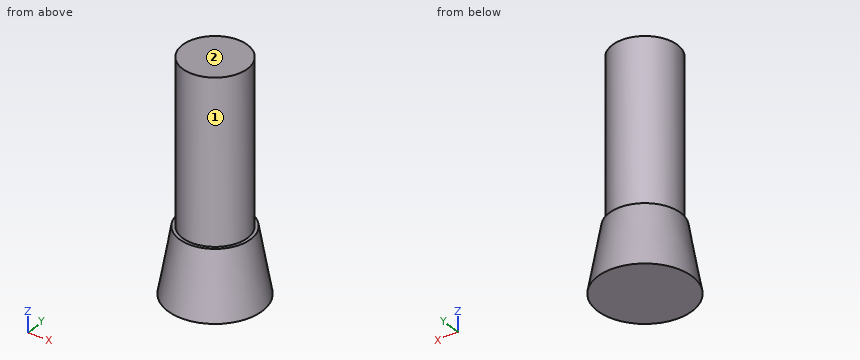
```python
from build123d import *

# Parameters (mm, degrees)
F0_R     = 12.7
F1_DEPTH = 88.9
F0_R_2   = 19.05
F2_DEPTH = 25.4


# Not quite as in the source:
# - a fillet or chamfer that OpenCascade refuses, or shapes differently, is made with other operations: its cross-section is extruded or revolved along the edge and cut away or added


with BuildPart() as f1:
    # F0 (on Top) → F1 (new body)
    with BuildSketch(Plane.XY):
        Circle(F0_R)
    extrude(amount=F1_DEPTH)

    # F0 (on Top) → F2 (join)
    with BuildSketch(Plane.XY):
        Circle(F0_R_2)
        Circle(F0_R, mode=Mode.SUBTRACT)
    extrude(amount=F2_DEPTH)

    # F3: chamfer of 5.08 x 28.8101116437 on 1 edges, made by hand

    # F3_s1 → F3_t2 (revolve, cut)
    with BuildSketch(Plane.XZ):
        Polygon((13.97, 25.4), (19.05, -3.4101116437), (19.05, 25.4), align=None)
    revolve(axis=Axis((0, 0, 25.4), (0, 0, 1)), mode=Mode.SUBTRACT)


solid = f1.part
```
For this review, take the finished solid that the model builds, in its own axes (mm). Face numbers are marked on the shaded views. A direction names the side the tool comes from. Round coordinates to 2 decimals unless told otherwise and drop trailing zeros. Write each loop counter-clockwise with the first axis right and the second up, starting at its lowest first coordinate (ties: lowest second). Pieces come first, ordered by that corner, then holes. Notation, with made-up numbers: (72, 30.5) -> (108, 30.5) arc R16 ccw to (108, 36.5) -> close; hole circle Ø7 at (23, 66). An arc over 180 degrees is marked (long way). One line per question, with ' | ' between items. Start each with the question number.
(1) Insertion check: P1, Ø5, axis at y = 5, z = 66, coming from the +X side; P2, Ø6, axis at x = 11.5, z = 46, coming from the +Y side; P3, Ø8, axis at x = 14.5, z = 32, coming from the -Y side. Each pin has a flat end and moves straight along its axis. Give the tip position at first contact, or say it passes through.
(2) Add section C-C, the plane z = 18. Write out the cut boundary in (x, y).
(3) For line 1 along Z through (x, y) = (-13, -1); line 2 along X through (y, z) = (2.5, 33); line 3 along X through (y, z) = (5.5, 54.5), list the stretches that pass through material, from the lowest coordinate up. Write a range as from..to.
(4) Tool access review of the marked faces 1 and 2: name each direction out of +Z, -Z, +X, -X, +Y, -Y from which nothing blocks a thin tool from reaching the whole face with its end or side.
(5) Add section A-A, the plane y = 0. Write out the cut boundary in (x, z), plus the area to 3 significant figures.
Answer list:
1) P1: x = 12.45 | P2: y = 9.44 | P3: y = -7.14
2) outline: circle Ø30.55 at (0, 0)
3) line 1: 0..25.4 | line 2: -12.45..12.45 | line 3: -11.45..11.45
4) face 1: +Z | face 2: +Z, +X, -X, +Y, -Y
5) outline: (-18.45, 0) -> (18.45, 0) -> (13.97, 25.4) -> (12.7, 25.4) -> (12.7, 88.9) -> (-12.7, 88.9) -> (-12.7, 25.4) -> (-13.97, 25.4) -> close | area: 2,440 mm²
